from build123d import *

# Parameters (mm, degrees)
SKETCH1_R                          = 31.5
BOSS_EXTRUDE1_DEPTH                = 22
TAP_DRILL_FOR_M3X0_5_TAP1_D        = 2.5
TAP_DRILL_FOR_M3X0_5_TAP1_DEPTH    = 4.76
TAP_DRILL_FOR_M3X0_5_TAP1_TIP      = 0.751075774
TAP_DRILL_FOR_M2_5X0_45_TAP1_D     = 2.05
TAP_DRILL_FOR_M2_5X0_45_TAP1_DEPTH = 3.5
TAP_DRILL_FOR_M2_5X0_45_TAP1_TIP   = 0.615882135
M2_5_CLEARANCE_HOLE1_D             = 2.9


with BuildPart() as part:
    # Sketch1 → Boss-Extrude1 (new body)
    with BuildSketch(Plane(origin=(0, 0, 0), x_dir=(1, 0, 0), z_dir=(0, 1, 0))):
        Circle(SKETCH1_R)
    extrude(amount=BOSS_EXTRUDE1_DEPTH)

    # Tap Drill for M3x0.5 Tap1
    with Locations(Plane(origin=(0, 22, 0), x_dir=(1, 0, 0), z_dir=(0, 1, 0))):
        with Locations((8.838834765, 8.838834765), (8.838834765, -8.838834765), (-8.838834765, -8.838834765), (-8.838834765, 8.838834765)):
            Hole(TAP_DRILL_FOR_M3X0_5_TAP1_D / 2, depth=TAP_DRILL_FOR_M3X0_5_TAP1_DEPTH)
            with Locations((0, 0, -(TAP_DRILL_FOR_M3X0_5_TAP1_DEPTH + TAP_DRILL_FOR_M3X0_5_TAP1_TIP / 2))):  # 118° drill point
                Cone(0, TAP_DRILL_FOR_M3X0_5_TAP1_D / 2, TAP_DRILL_FOR_M3X0_5_TAP1_TIP, mode=Mode.SUBTRACT)

    # Tap Drill for M2.5x0.45 Tap1
    with Locations(Plane(origin=(0, 0, 0), x_dir=(-1, 0, 0), z_dir=(0, -1, 0))):
        with Locations((5.303300859, -5.303300859), (5.303300859, 5.303300859), (-5.303300859, -5.303300859), (-5.303300859, 5.303300859)):
            Hole(TAP_DRILL_FOR_M2_5X0_45_TAP1_D / 2, depth=TAP_DRILL_FOR_M2_5X0_45_TAP1_DEPTH)
            with Locations((0, 0, -(TAP_DRILL_FOR_M2_5X0_45_TAP1_DEPTH + TAP_DRILL_FOR_M2_5X0_45_TAP1_TIP / 2))):  # 118° drill point
                Cone(0, TAP_DRILL_FOR_M2_5X0_45_TAP1_D / 2, TAP_DRILL_FOR_M2_5X0_45_TAP1_TIP, mode=Mode.SUBTRACT)

    # M2.5 Clearance Hole1 (through all)
    with Locations(Plane(origin=(0, 22, 0), x_dir=(1, 0, 0), z_dir=(0, 1, 0))):
        with Locations((5.303300859, 5.303300859), (5.303300859, -5.303300859), (-5.303300859, -5.303300859), (-5.303300859, 5.303300859)):
            Hole(M2_5_CLEARANCE_HOLE1_D / 2)


solid = part.part
The listing builds one solid part. Answer for the finished solid, in the listing's coordinates (mm). A direction names the side the tool comes from. Round coordinates to 2 decimals unless told otherwise and drop trailing zeros. Write each loop counter-clockwise with the first axis right and the second up, starting at its lowest first coordinate (ties: lowest second). Pieces come first, ordered by that corner, then holes. Notation, with made-up numbers: (-36.75, 5) - (-10.75, 5) arc R9 cw to (-10.75, 18) - close; hole circle Ø2 at (-40, 47.25). An arc over 180 degrees is marked (long way). Use a Markdown table: item, result. Add a question column.
1. For a pull along Z with two mould halves and no side action, classify faces 3 (the face through (-4.101, 10.846, -31.232)), 4 (the face through (8.79, 16.62, 9.05)), 5 (the face through (0, 22, 0)) as +Z half, -Z half, draft (parallel to the pull), parting line (faces both ways), or undercut.
2. The part is cut by section B-B (x = 26.5). Write down the section's boundary in (y, z), and give its area (3 significant figures).
3. A tool of negligible diameter and unlimited length cuts with its end or side. For faces 1 (the face through (5.62, 10.85, -3.89)), 2 (the face through (-7.59, 19.59, 8.78)), from which of +Z, -Z, +X, -X, +Y, -Y can it reach the whole face along a straight path? Write none if from no direction.
4. Flat-ended cylindrical pins translate along their axes: P1, Ø2.5, axis at x = 5.3, z = 5.3, coming from the +Y side; P2, Ø2, axis at x = 8.84, z = 8.84, coming from the +Y side; P3, Ø1, axis at y = 18, z = -6, coming from the +X side; P4, Ø2, axis at x = -14.5, y = 6.5, coming from the -Z side. Find the tip coordinate at first contact, or state that the pin passes through.
5. Consider line 1 (X direction, y = 17, z = -4.5); line 2 (X direction, y = 13, z = -5). Determine where each line is inside the solid, lowest interval first.
6. The part is cut by section C-C (z = -16.5). Write down the section's boundary in (x, y).
7. The part is cut by section A-A (y = 3.25). Write down the section's boundary in (x, z), and give its area (3 significant figures).
Reported:
| question | item | result |
|---|---|---|
| 1 | face 3 | parting line |
| 1 | face 4 | undercut |
| 1 | face 5 | draft |
| 2 | outline | (0, -17.03) - (22, -17.03) - (22, 17.03) - (0, 17.03) - close |
| 2 | area | 749 mm^2 |
| 3 | face 1 | +Y, -Y |
| 3 | face 2 | +Y |
| 4 | P1 | through |
| 4 | P2 | y = 17.09 |
| 4 | P3 | x = 31.02 |
| 4 | P4 | z = -28.46 |
| 5 | line 1 | -31.18 to -6.51, -4.1 to 4.1, 6.51 to 31.18 |
| 5 | line 2 | -31.1 to -6.72, -3.89 to 3.89, 6.72 to 31.1 |
| 6 | outline | (-26.83, 0) - (26.83, 0) - (26.83, 22) - (-26.83, 22) - close |
| 7 | outline | circle Ø63 at (0, 0); hole circle Ø2.9 at (-5.3, -5.3); hole circle Ø2.9 at (-5.3, 5.3); hole circle Ø2.9 at (5.3, -5.3); hole circle Ø2.9 at (5.3, 5.3) |
| 7 | area | 3,090 mm^2 |
